Read the model definition and answer for the solid it produces. Units are mm, in the model's axes. Face numbers are marked on the shaded views. A direction names the side the tool comes from. Round coordinates to 2 decimals unless told otherwise and drop trailing zeros. Order: outer loops, then holes, each group sorted by start corner. A loop starts at its lowest first (then second) coordinate and runs counter-clockwise, first axis right, second up. Notation, with made-up numbers: (-9, 74) - (1, 74) arc R20 ccw to (1, 86) - close; hole circle Ø8 at (79.5, 7). An arc over 180 degrees is marked (long way). Put each result on its own line as item: value. Start each with the question number.
Q1. Which of the six approach directions +Z, -Z, +X, -X, +Y, -Y give full straight-line access (tool end or side, diameter ignored) to the marked faces 4, 5 and 6?
Q2. Section A-A on z = 8 is taken. Give the vertices of the cut face in (x, y).
Q3. For a pull along Z with two mould halves and no side action, classify the marked faces 1, 2 and 3 as pulls with the +Z half, pulls with the -Z half, needs draft (parallel to the pull), parting line crosses it, or undercut.
Q4. Section D-D on z = 20 is taken. Give the vertices of the cut face in (x, y).
Q5. Section B-B on z = 32 is taken. State how many separate pieces and enclosed holes the cut face has, then the cut area to 3 significant figures.
Q6. Find the intervals of material crossed by line 1 along Z through (x, y) = (-78, 25.25); line 2 along X through (y, z) = (30.25, 20); line 3 along X through (y, z) = (19.25, 33), in increasing order. Write a range as from..to.
Q7. Each of these flat-tipped pins is pushed along its axis until it touches: pin 1 Ø13 at (x, z) = (-78.07, 32) entering from -Y; pin 2 Ø11 at (x, z) = (-51, 32.5) entering from +Y; pin 3 Ø6 at (x, z) = (-22.07, 32) entering from +Y. Where does it stop, or does it pass through?
from build123d import *

# Parameters (mm, degrees)
AUFSATZ_LINEAR_AUSTRAGEN1_DEPTH  = 40
DURCHGANGSLOCH_F_R_M41_D         = 4.3
DURCHGANGSLOCH_F_R_M42_D         = 4.3
F_5_3_5_3_DURCHMESSER_BOHRUNG1_D = 5.3
DURCHGANGSLOCH_F_R_M81_D         = 8.4
SKIZZE26_R                       = 5
SCHNITT_LINEAR_AUSTRAGEN3_DEPTH  = 12
SKIZZE27_R                       = 5
SCHNITT_LINEAR_AUSTRAGEN4_DEPTH  = 7


with BuildPart() as part:
    # Skizze1 → Aufsatz-Linear austragen1 (new body)
    with BuildSketch(Plane.XY):
        Polygon((-85.072105864, 34.368747103), (-85.072105864, 14.368747103), (-50.072105864, 14.368747103), (-50.072105864, 28.368747103), (-65.805439197, 28.368747103), (-65.805439197, 34.368747103), align=None)
        Polygon((-50.072105864, 28.368747103), (-50.072105864, 14.368747103), (-15.072105864, 14.368747103), (-15.072105864, 34.368747103), (-34.33877253, 34.368747103), (-34.33877253, 28.368747103), align=None)
    extrude(amount=AUFSATZ_LINEAR_AUSTRAGEN1_DEPTH)

    # Durchgangsloch für M41 (through all)
    with Locations(Plane(origin=(0, 28.368747103, 0), x_dir=(1, 0, 0), z_dir=(0, 1, 0))):
        with Locations((-50.072105864, -8)):
            Hole(DURCHGANGSLOCH_F_R_M41_D / 2)

    # Durchgangsloch für M42 (through all)
    with Locations(Plane(origin=(0, 34.368747103, 0), x_dir=(1, 0, 0), z_dir=(0, 1, 0))):
        with Locations((-78.072105864, -5), (-78.072105864, -20), (-22.072105864, -20), (-22.072105864, -5)):
            Hole(DURCHGANGSLOCH_F_R_M42_D / 2)

    # Ø5.3 (5.3) Durchmesser Bohrung1 (through all)
    with Locations(Plane(origin=(0, 34.368747103, 0), x_dir=(1, 0, 0), z_dir=(0, 1, 0))):
        with Locations((-78.072105864, -32), (-22.072105864, -32)):
            Hole(F_5_3_5_3_DURCHMESSER_BOHRUNG1_D / 2)

    # Durchgangsloch für M81 (through all)
    with Locations(Plane(origin=(0, 28.368747103, 0), x_dir=(1, 0, 0), z_dir=(0, 1, 0))):
        with Locations((-50.072105864, -32)):
            Hole(DURCHGANGSLOCH_F_R_M81_D / 2)

    # Skizze26 → Schnitt-Linear austragen3 (cut)
    with BuildSketch(Plane(origin=(0, 34.368747103, 0), x_dir=(1, 0, 0), z_dir=(0, 1, 0))):
        with Locations((-78.072105864, -32)):
            Circle(SKIZZE26_R)
        with Locations((-22.072105864, -32)):
            Circle(SKIZZE26_R)
    extrude(amount=-SCHNITT_LINEAR_AUSTRAGEN3_DEPTH, mode=Mode.SUBTRACT)

    # Skizze27 → Schnitt-Linear austragen4 (cut)
    with BuildSketch(Plane(origin=(0, 28.368747103, 0), x_dir=(1, 0, 0), z_dir=(0, 1, 0))):
        with Locations((-50.072105864, -32)):
            Circle(SKIZZE27_R)
    extrude(amount=-SCHNITT_LINEAR_AUSTRAGEN4_DEPTH, mode=Mode.SUBTRACT)


solid = part.part
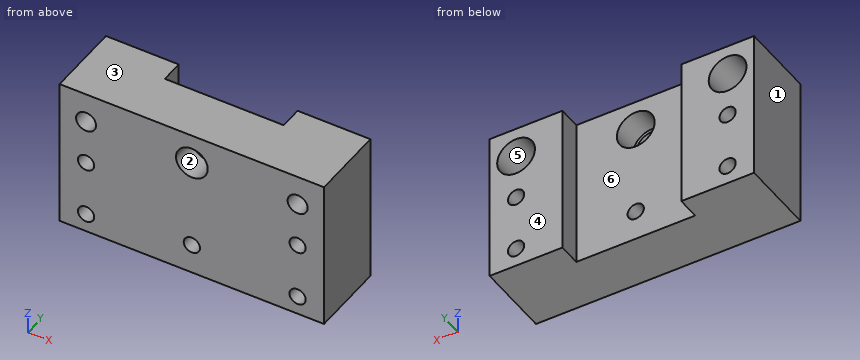
Findings:
1. face 4: +Z, -Z, +X, -X, +Y
1. face 5: +Y
1. face 6: +Z, -Z, +Y
2. outline: (-85.07, 14.37) - (-52.22, 14.37) - (-52.22, 28.37) - (-65.81, 28.37) - (-65.81, 34.37) - (-85.07, 34.37) - close; (-47.92, 14.37) - (-15.07, 14.37) - (-15.07, 34.37) - (-34.34, 34.37) - (-34.34, 28.37) - (-47.92, 28.37) - close
3. face 1: needs draft
3. face 2: undercut
3. face 3: pulls with the +Z half
4. outline: (-85.07, 14.37) - (-80.22, 14.37) - (-80.22, 34.37) - (-85.07, 34.37) - close; (-75.92, 14.37) - (-24.22, 14.37) - (-24.22, 34.37) - (-34.34, 34.37) - (-34.34, 28.37) - (-65.81, 28.37) - (-65.81, 34.37) - (-75.92, 34.37) - close; (-19.92, 14.37) - (-15.07, 14.37) - (-15.07, 34.37) - (-19.92, 34.37) - close
5. separate pieces: 4
5. enclosed holes: 0
5. area: 758 mm2
6. line 1: 0..2.85, 7.15..17.85, 22.15..27, 37..40
6. line 2: -85.07..-80.22, -75.92..-65.81, -34.34..-24.22, -19.92..-15.07
6. line 3: -85.07..-80.53, -75.62..-54.15, -45.99..-24.53, -19.62..-15.07
7. pin 1: y = 14.37
7. pin 2: y = 28.37
7. pin 3: y = 22.37
